Work out the finished part from the listing and answer in its coordinate system (mm). A direction names the side the tool comes from. Give positions to 0.01 mm unless a question says otherwise; leave off trailing zeros. Order: outer loops, then holes, each group sorted by start corner. A loop starts at its lowest first (then second) coordinate and runs counter-clockwise, first axis right, second up. Notation, with made-up numbers: (8, -1.5) - (21, -1.5) arc R28 ccw to (21, 28.5) - close; hole circle Ø2 at (-15.75, 63.5). An arc over 180 degrees is marked (long way). Write each question's results on one line, items separated by ' | '.
from build123d import *

# Parameters (mm, degrees)
SKETCH1_W                   = 116
SKETCH1_H                   = 116
BOSS_EXTRUDE1_DEPTH         = 2
CUT_EXTRUDE1_REACH          = 84.049
SKETCH2_W                   = 15
SKETCH2_H                   = 76
CIRPATTERN1_COUNT           = 2
CUT_EXTRUDE2_REACH          = 84.049
SKETCH3_R                   = 1.5
CUT_EXTRUDE3_REACH          = 84.049
SKETCH4_R                   = 1.5
LPATTERN1_COUNT             = 2
LPATTERN1_PITCH             = 23
CIRPATTERN2_COUNT           = 2
CIRPATTERN2_COPY_1_REACH    = 84.049
CIRPATTERN2_COPY_1_SKETCH_R = 1.5
CIRPATTERN2_COPY_2_REACH    = 84.049
CIRPATTERN2_COPY_2_SKETCH_R = 1.5
CUT_EXTRUDE4_REACH          = 84.049
SKETCH5_W                   = 76
SKETCH5_H                   = 16
SKETCH6_W                   = 6
SKETCH6_H                   = 4
BOSS_EXTRUDE2_DEPTH         = 6
CUT_EXTRUDE5_REACH          = 131.938
SKETCH7_R                   = 1.5
CUT_EXTRUDE7_REACH          = 84.244
SKETCH9_W                   = 5
SKETCH9_H                   = 76
BOSS_EXTRUDE3_DEPTH         = 1.5
SKETCH10_W                  = 76
SKETCH10_H                  = 3
BOSS_EXTRUDE4_DEPTH         = 3.5
SKETCH11_W                  = 2.5
SKETCH11_H                  = 14.264665063
BOSS_EXTRUDE5_DEPTH         = 1.5


with BuildPart() as part:
    # Sketch1 → Boss-Extrude1 (new body)
    with BuildSketch(Plane(origin=(0, 0, 0), x_dir=(1, 0, 0), z_dir=(0, 1, 0))):
        Rectangle(SKETCH1_W, SKETCH1_H)
    extrude(amount=BOSS_EXTRUDE1_DEPTH)

    # Sketch2 → Cut-Extrude1 (cut, up to next)
    with BuildSketch(Plane(origin=(0, 2, 0), x_dir=(1, 0, 0), z_dir=(0, 1, 0)), mode=Mode.PRIVATE) as cut_extrude1_sk1:
        with Locations((-50.5, 0)):
            Rectangle(SKETCH2_W, SKETCH2_H)
    cut_extrude1_tool1 = extrude(cut_extrude1_sk1.sketch, amount=-CUT_EXTRUDE1_REACH, mode=Mode.PRIVATE) & part.part
    cut_extrude1 = cut_extrude1_tool1.solids().sort_by_distance((-50.5, 2, 0))[0]
    add(cut_extrude1, mode=Mode.SUBTRACT)

    # CirPattern1: Cut-Extrude1 ×2 about axis
    cirpattern1_axis = Axis((0, 0, 0), (0, 1, 0))
    for i in range(1, CIRPATTERN1_COUNT):
        add(cut_extrude1.rotate(cirpattern1_axis, i * 360 / CIRPATTERN1_COUNT), mode=Mode.SUBTRACT)

    # Sketch3 → Cut-Extrude2 (cut, up to next)
    with BuildSketch(Plane(origin=(0, 2, 0), x_dir=(1, 0, 0), z_dir=(0, 1, 0)), mode=Mode.PRIVATE) as cut_extrude2_sk1:
        with Locations(Location((-29, 37, 0), (0, 0, 270))):
            Circle(SKETCH3_R)
    cut_extrude2_tool1 = extrude(cut_extrude2_sk1.sketch, amount=-CUT_EXTRUDE2_REACH, mode=Mode.PRIVATE) & part.part
    cut_extrude2 = cut_extrude2_tool1.solids().sort_by_distance((-29, 2, -37))[0]
    add(cut_extrude2, mode=Mode.SUBTRACT)

    # Sketch4 → Cut-Extrude3 (cut, up to next)
    with BuildSketch(Plane(origin=(0, 2, 0), x_dir=(1, 0, 0), z_dir=(0, 1, 0)), mode=Mode.PRIVATE) as cut_extrude3_sk1:
        with Locations(Location((29, 37, 0), (0, 0, 270))):
            Circle(SKETCH4_R)
    cut_extrude3_tool1 = extrude(cut_extrude3_sk1.sketch, amount=-CUT_EXTRUDE3_REACH, mode=Mode.PRIVATE) & part.part
    cut_extrude3 = cut_extrude3_tool1.solids().sort_by_distance((29, 2, -37))[0]
    add(cut_extrude3, mode=Mode.SUBTRACT)

    # LPattern1: Cut-Extrude2, Cut-Extrude3 ×2
    with Locations(*[(0, 0, i * LPATTERN1_PITCH) for i in range(1, LPATTERN1_COUNT)]):
        add(cut_extrude2, mode=Mode.SUBTRACT)
        add(cut_extrude3, mode=Mode.SUBTRACT)

    # CirPattern2: Cut-Extrude2, Cut-Extrude3 ×2 about axis
    cirpattern2_axis = Axis((0, 0, 0), (0, 1, 0))
    add([cut_extrude2.rotate(cirpattern2_axis, i * 360 / CIRPATTERN2_COUNT) for i in range(1, CIRPATTERN2_COUNT)], mode=Mode.SUBTRACT)
    add([cut_extrude3.rotate(cirpattern2_axis, i * 360 / CIRPATTERN2_COUNT) for i in range(1, CIRPATTERN2_COUNT)], mode=Mode.SUBTRACT)

    # CirPattern2 copy 1 sketch → CirPattern2 copy 1 (cut, up to next)
    with BuildSketch(Plane(origin=(0, 2, -23), x_dir=(-1, 0, 0), z_dir=(0, 1, 0)), mode=Mode.PRIVATE) as cirpattern2_copy_1_sk1:
        with Locations(Location((-29, 37, 0), (0, 0, 270))):
            Circle(CIRPATTERN2_COPY_1_SKETCH_R)
    cirpattern2_copy_1_tool1 = extrude(cirpattern2_copy_1_sk1.sketch, amount=-CIRPATTERN2_COPY_1_REACH, mode=Mode.PRIVATE) & part.part
    add(cirpattern2_copy_1_tool1.solids().sort_by_distance((29, 2, 14))[0], mode=Mode.SUBTRACT)

    # CirPattern2 copy 2 sketch → CirPattern2 copy 2 (cut, up to next)
    with BuildSketch(Plane(origin=(0, 2, -23), x_dir=(-1, 0, 0), z_dir=(0, 1, 0)), mode=Mode.PRIVATE) as cirpattern2_copy_2_sk1:
        with Locations(Location((29, 37, 0), (0, 0, 270))):
            Circle(CIRPATTERN2_COPY_2_SKETCH_R)
    cirpattern2_copy_2_tool1 = extrude(cirpattern2_copy_2_sk1.sketch, amount=-CIRPATTERN2_COPY_2_REACH, mode=Mode.PRIVATE) & part.part
    add(cirpattern2_copy_2_tool1.solids().sort_by_distance((-29, 2, 14))[0], mode=Mode.SUBTRACT)

    # Sketch5 → Cut-Extrude4 (cut, up to next)
    with BuildSketch(Plane(origin=(0, 2, 0), x_dir=(1, 0, 0), z_dir=(0, 1, 0)), mode=Mode.PRIVATE) as cut_extrude4_sk1:
        Rectangle(SKETCH5_W, SKETCH5_H)
    cut_extrude4_tool1 = extrude(cut_extrude4_sk1.sketch, amount=-CUT_EXTRUDE4_REACH, mode=Mode.PRIVATE) & part.part
    add(cut_extrude4_tool1.solids().sort_by_distance((0, 2, 0))[0], mode=Mode.SUBTRACT)

    # Sketch6 → Boss-Extrude2 (add)
    with BuildSketch(Plane(origin=(0, 2, 0), x_dir=(1, 0, 0), z_dir=(0, 1, 0))):
        with Locations((45, -56)):
            Rectangle(SKETCH6_W, SKETCH6_H)
    boss_extrude2 = extrude(amount=BOSS_EXTRUDE2_DEPTH)

    # Sketch7 → Cut-Extrude5 (cut, up to next)
    with BuildSketch(Plane.XY.offset(58), mode=Mode.PRIVATE) as cut_extrude5_sk1:
        with Locations((45, 5)):
            Circle(SKETCH7_R)
    cut_extrude5_tool1 = extrude(cut_extrude5_sk1.sketch, amount=-CUT_EXTRUDE5_REACH, mode=Mode.PRIVATE) & part.part
    cut_extrude5 = cut_extrude5_tool1.solids().sort_by_distance((45, 5, 58))[0]
    add(cut_extrude5, mode=Mode.SUBTRACT)

    # Mirror1: Boss-Extrude2, Cut-Extrude5 across plane
    add(boss_extrude2.mirror(Plane.XY))
    add(cut_extrude5.mirror(Plane.XY), mode=Mode.SUBTRACT)

    # Sketch8 → Cut-Extrude7 (cut, up to next)
    with BuildSketch(Plane(origin=(0, 2, 0), x_dir=(1, 0, 0), z_dir=(0, 1, 0)), mode=Mode.PRIVATE) as cut_extrude7_sk1:
        with BuildLine():
            ThreePointArc((-29, -33.5), (-26.525126266, -34.525126266), (-25.5, -37))
            Line((-25.5, -37), (25.5, -37))
            ThreePointArc((25.5, -37), (26.525126266, -34.525126266), (29, -33.5))
            Line((29, -33.5), (29, -17.5))
            ThreePointArc((29, -17.5), (26.525126266, -16.474873734), (25.5, -14))
            Line((25.5, -14), (-25.5, -14))
            ThreePointArc((-25.5, -14), (-26.525126266, -16.474873734), (-29, -17.5))
            Line((-29, -17.5), (-29, -33.5))
        make_face()
    cut_extrude7_tool1 = extrude(cut_extrude7_sk1.sketch, amount=-CUT_EXTRUDE7_REACH, mode=Mode.PRIVATE) & part.part
    cut_extrude7 = cut_extrude7_tool1.solids().sort_by_distance((0, 2, 25.5))[0]
    add(cut_extrude7, mode=Mode.SUBTRACT)

    # Mirror2: Cut-Extrude7 across plane
    add(cut_extrude7.mirror(Plane.XY), mode=Mode.SUBTRACT)

    # Sketch9 → Boss-Extrude3 (add)
    with BuildSketch(Plane(origin=(0, 2, 0), x_dir=(1, 0, 0), z_dir=(0, 1, 0))):
        with Locations((-40.5, 0)):
            Rectangle(SKETCH9_W, SKETCH9_H)
    boss_extrude3 = extrude(amount=BOSS_EXTRUDE3_DEPTH)

    # Mirror3: Boss-Extrude3 across plane
    add(boss_extrude3.mirror(Plane(origin=(0, 0, 0), x_dir=(0, 0, 1), z_dir=(1, 0, 0))))

    # Sketch10 → Boss-Extrude4 (add)
    with BuildSketch(Plane(origin=(0, 0, 0), x_dir=(-1, 0, 0), z_dir=(0, -1, 0))):
        with Locations((0, 6.5)):
            Rectangle(SKETCH10_W, SKETCH10_H)
    boss_extrude4 = extrude(amount=-BOSS_EXTRUDE4_DEPTH)

    # Mirror4: Boss-Extrude4 across plane
    add(boss_extrude4.mirror(Plane.XY))

    # Sketch11 → Boss-Extrude5 (add)
    with BuildSketch(Plane(origin=(0, 2, 0), x_dir=(1, 0, 0), z_dir=(0, 1, 0))):
        with Locations((26.25, -50.867667469)):
            Rectangle(SKETCH11_W, SKETCH11_H)
    boss_extrude5 = extrude(amount=BOSS_EXTRUDE5_DEPTH)

    # Mirror5: Boss-Extrude5 across plane
    add(boss_extrude5.mirror(Plane.XY))


solid = part.part
1. A tool of negligible diameter and unlimited length cuts with its end or side. For faces 5 (the face through (43, 2, 1)), 6 (the face through (-43, 2, 1)), 7 (the face through (43.6, 3.6, -54)), 8 (the face through (48, 5, 56)), 9 (the face through (-26.5, 1.01, -16.45)), from which of +Z, -Z, +X, -X, +Y, -Y can it reach the whole face along a straight path? Write none if from no direction.
Answer list:
face 5: +X, +Y, -Y | face 6: -X, +Y, -Y | face 7: +X, +Y | face 8: +Z, -Z, +X, +Y | face 9: +Y, -Y
2. A cutting plane is placed at B-B, the plane z = -32. Write down the section's boundary in (x, y), then the cut area to 3 significant figures.
Answer list:
outline: (-43, 0) - (-29, 0) - (-29, 2) - (-38, 2) - (-38, 3.5) - (-43, 3.5) - close; (29, 0) - (43, 0) - (43, 3.5) - (38, 3.5) - (38, 2) - (29, 2) - close | area: 71.0 mm^2
3. Given P1, Ø1.2, axis at y = 3, z = 47.5, coming from the +X side; P2, Ø1.5, axis at x = 44.5, z = -32, coming from the -Y side; P3, Ø0.6, axis at y = 1.5, z = 29, coming from the -X side; P4, Ø3.5, axis at x = 29, z = 37, coming from the -Y side, each flat-ended and moving along its own axis, determine where each tip first touches the part or whether it passes through.
Answer list:
P1: x = 27.5 | P2: through | P3: x = -43 | P4: y = 0
4. A cutting plane is placed at A-A, the plane x = 21. Write down the section's boundary in (y, z), then the cut area to 3 significant figures.
Answer list:
outline: (0, -58) - (2, -58) - (2, -37) - (0, -37) - close; (0, -14) - (2, -14) - (2, -8) - (3.5, -8) - (3.5, -5) - (0, -5) - close; (0, 5) - (3.5, 5) - (3.5, 8) - (2, 8) - (2, 14) - (0, 14) - close; (0, 37) - (2, 37) - (2, 58) - (0, 58) - close | area: 129 mm^2
5. Determine the mould class of faces 1 (the face through (27.99, 1.01, 15.11)), 2 (the face through (-27.513, 1.014, -14.195)), 3 (the face through (48, 5, -56)), 4 (the face through (8, 1, 58)) for opening direction Z: +Z half, -Z half, draft (parallel to the pull), parting line (faces both ways), or undercut.
Answer list:
face 1: undercut | face 2: undercut | face 3: draft | face 4: +Z half
6. A cutting plane is placed at D-D, the plane x = 45. Write down the section's boundary in (y, z).
Answer list:
outline: (0, -58) - (3.5, -58) - (3.5, -54) - (2, -54) - (2, -38) - (0, -38) - close; (0, 38) - (2, 38) - (2, 54) - (3.5, 54) - (3.5, 58) - (0, 58) - close; (6.5, -58) - (8, -58) - (8, -54) - (6.5, -54) - close; (6.5, 54) - (8, 54) - (8, 58) - (6.5, 58) - close
7. A cutting plane is placed at C-C, the plane z = -47. Write down the section's boundary in (x, y).
Answer list:
outline: (-58, 0) - (58, 0) - (58, 2) - (27.5, 2) - (27.5, 3.5) - (25, 3.5) - (25, 2) - (-58, 2) - close
8. Straight lines are drawn through the part: line 1 (Z direction, x = 15.5, y = 0.75); line 2 (Y direction, x = 45, z = 56.85); line 3 (Z direction, x = 10, y = 2.25). For each, find the intervals that lie inside material, in ascending order. Write a range as [from, to].
Answer list:
line 1: [-58, -37], [-14, -5], [5, 14], [37, 58] | line 2: [0, 3.5], [6.5, 8] | line 3: [-8, -5], [5, 8]
